Verification items for the finished model (mm, model axes). A direction names the side the tool comes from. Round coordinates to 2 decimals unless told otherwise and drop trailing zeros. Order: outer loops, then holes, each group sorted by start corner. A loop starts at its lowest first (then second) coordinate and runs counter-clockwise, first axis right, second up. Notation, with made-up numbers: (54, 24) -> (105, 24) arc R20 cw to (105, 35) -> close; hole circle Ø2 at (-17, 43). An arc over 180 degrees is marked (long way). Write item = value, one per line. Start each with the question number.
from build123d import *

# Parameters (mm, degrees)
F1_DEPTH = 44.45
F2_R     = 3.175
F3_W     = 19.05
F3_H     = 50.8
F4_DEPTH = 50.801
F5_SIZE  = 5.08


with BuildPart() as f1:
    # F0 (on Front) → F1 (new body)
    with BuildSketch(Plane.XZ):
        with BuildLine():
            ThreePointArc((25.4, 53.975), (20.75032, 65.20032), (9.525, 69.85))
            Line((9.525, 69.85), (-9.525, 69.85))
            ThreePointArc((-9.525, 69.85), (-20.75032, 65.20032), (-25.4, 53.975))
            Line((-25.4, 53.975), (-25.4, -53.975))
            ThreePointArc((-25.4, -53.975), (-20.75032, -65.20032), (-9.525, -69.85))
            Line((-9.525, -69.85), (9.525, -69.85))
            ThreePointArc((9.525, -69.85), (20.75032, -65.20032), (25.4, -53.975))
            Line((25.4, -53.975), (25.4, 53.975))
        make_face()
    extrude(amount=F1_DEPTH)

    # F2
    f2_edges = [f1.edges().sort_by_distance(p)[0] for p in [
        (20.75032, -44.45, 65.20032),
        (0, -44.45, 69.85),
        (-20.75032, -44.45, 65.20032),
        (-25.4, -44.45, 0),
        (-20.75032, -44.45, -65.20032),
        (0, -44.45, -69.85),
        (20.75032, -44.45, -65.20032),
        (25.4, -44.45, 0),
        (20.75032, 0, 65.20032),
        (0, 0, 69.85),
        (-20.75032, 0, 65.20032),
        (-25.4, 0, 0),
        (-20.75032, 0, -65.20032),
        (0, 0, -69.85),
        (20.75032, 0, -65.20032),
        (25.4, 0, 0),
    ]]
    fillet(f2_edges, radius=F2_R)

    # F3 (on face) → F4 (cut, through all)
    with BuildSketch(Plane.YZ.offset(25.4)):
        with Locations((-22.225, 0)):
            Rectangle(F3_W, F3_H)
    extrude(amount=-F4_DEPTH, mode=Mode.SUBTRACT)

    # F5
    f5_edges = [f1.edges().sort_by_distance(p)[0] for p in [
        (25.4, -31.75, 0),
        (25.4, -22.225, 25.4),
        (25.4, -12.7, 0),
        (25.4, -22.225, -25.4),
        (-25.4, -22.225, 25.4),
        (-25.4, -31.75, 0),
        (-25.4, -22.225, -25.4),
        (-25.4, -12.7, 0),
    ]]
    chamfer(f5_edges, length=F5_SIZE)


solid = f1.part
(1) Cross-section at B-B (x = 0.5). Enter the section's corners in (y, z) (3 decimals), and give its area (3 significant figures).
(2) Set-up check for faces 1 (the cylindrical face through (24.49, -0.95, 0.76)), 2 (the flat face through (-22.9, -10.12, -0.43)), 3 (the flat face through (22.82, -10.2, -0.43)): record each of +Z, -Z, +X, -X, +Y, -Y from which the full face is reachable in a straight line by a thin tool's end or side.
(3) Cross-section at C-C (z = -15.5). Enter the section's corners in (x, y) (3 decimals), and give its area (3 significant figures).
(4) Draft check along Z on faces 4 (the flat face through (0, 0, 1)), 5 (the cylindrical face through (0.13, -0.95, -68.94)), 6 (the flat face through (-22.9, -34.33, -0.43)). Enter one of: +Z half, -Z half, draft (parallel to the pull), parting line (faces both ways), or undercut.
(5) Scan lines: line 1 along Y through (x, z) = (-10, -17); line 2 along Z through (x, y) = (4.5, -28); line 3 along Z through (x, y) = (12.5, -29). Record each from-to range of solid material in increasing order. Write a range as from..to.
(6) Cross-section at A-A (y = -17.5). Enter the section's corners in (x, z) (3 decimals).
(7) Depth check by flat-ended pin: pin 1 (10 mm diameter, centred on y = -14.5, z = -2.5, fed in from +X); pin 2 (3 mm diameter, centred on y = -10.5, z = -10.5, fed in from +X); pin 3 (1 mm diameter, centred on x = 10.5, y = -6.5, fed in from +Z). Enter the tip coordinate at first touch or a pass-through.
Outcome:
q1.outline = (-44.45, -66.675) arc R3.175 ccw to (-41.275, -69.85) -> (-3.175, -69.85) arc R3.175 ccw to (0, -66.675) -> (0, 66.675) arc R3.175 ccw to (-3.175, 69.85) -> (-41.275, 69.85) arc R3.175 ccw to (-44.45, 66.675) -> close; hole (-31.75, -25.4) -> (-12.7, -25.4) -> (-12.7, 25.4) -> (-31.75, 25.4) -> close
q1.area = 5,230 mm^2
q2.face_1 = +Z, -Z, +X, +Y
q2.face_2 = -X
q2.face_3 = +X
q3.outline = (-25.4, -41.275) arc R3.175 ccw to (-22.225, -44.45) -> (22.225, -44.45) arc R3.175 ccw to (25.4, -41.275) -> (25.4, -36.83) -> (20.32, -31.75) -> (-20.32, -31.75) -> (-25.4, -36.83) -> close; (-25.4, -7.62) -> (-20.32, -12.7) -> (20.32, -12.7) -> (25.4, -7.62) -> (25.4, -3.175) arc R3.175 ccw to (22.225, 0) -> (-22.225, 0) arc R3.175 ccw to (-25.4, -3.175) -> close
q3.area = 1,230 mm^2
q4.face_4 = draft
q4.face_5 = -Z half
q4.face_6 = undercut
q5.line_1 = -44.45..-31.75, -12.7..0
q5.line_2 = -69.85..-25.4, 25.4..69.85
q5.line_3 = -69.57..-25.4, 25.4..69.57
q6.outline = (-25.4, -53.975) arc R15.875 ccw to (-9.525, -69.85) -> (9.525, -69.85) arc R15.875 ccw to (25.4, -53.975) -> (25.4, -30.48) -> (20.32, -25.4) -> (-20.32, -25.4) -> (-25.4, -30.48) -> close; (-25.4, 30.48) -> (-20.32, 25.4) -> (20.32, 25.4) -> (25.4, 30.48) -> (25.4, 53.975) arc R15.875 ccw to (9.525, 69.85) -> (-9.525, 69.85) arc R15.875 ccw to (-25.4, 53.975) -> close
q7.pin_1 = 23.52
q7.pin_2 = 24.02
q7.pin_3 = 69.84
